```python
from build123d import *

# Parameters (mm, degrees)
F0_W     = 53
F0_H     = 10
F0_R     = 1.8
F1_DEPTH = 8
F2_R     = 1.8
F3_DEPTH = 5
F4_R     = 3


with BuildPart() as f1:
    # F0 (on Front) → F1 (new body)
    with BuildSketch(Plane.XZ):
        with Locations((-26.5, 5)):
            Rectangle(F0_W, F0_H)
        with Locations((-48.5, 5)):
            Circle(F0_R, mode=Mode.SUBTRACT)
        with Locations((-4.5, 5)):
            Circle(F0_R, mode=Mode.SUBTRACT)
        with Locations((-48.5, 5)):
            Circle(F0_R)
        with Locations((-4.5, 5)):
            Circle(F0_R)
    extrude(amount=F1_DEPTH)

    # F2 (on face) → F3 (cut)
    with BuildSketch(Plane(origin=(0, 0, 0), x_dir=(-1, 0, 0), z_dir=(0, 1, 0))):
        with Locations((4.5, 5)):
            Circle(F2_R)
        with Locations((48.5, 5)):
            Circle(F2_R)
    extrude(amount=-F3_DEPTH, mode=Mode.SUBTRACT)

    # F4
    f4_edges = [f1.edges().sort_by_distance(p)[0] for p in [
        (0, -4, 10),
        (0, -4, 0),
        (-53, -4, 10),
        (-53, -4, 0),
    ]]
    fillet(f4_edges, radius=F4_R)


solid = f1.part
```
Geometry: final body of the model. Coordinates: model frame, mm. A direction names the side the tool comes from. Give positions to 0.01 mm unless a question says otherwise; leave off trailing zeros. Loops run counter-clockwise (first coordinate to the right, second up) from the corner with the lowest first, then second, coordinate; pieces in that order, holes last. Notation, with made-up numbers: (35, 27) -> (52, 27) arc R28 ccw to (52, 62) -> close; hole circle Ø7 at (31, 36). An arc over 180 degrees is marked (long way). Return JSON: item names as keys, results as strings.
Item 1: Section C-C, the plane x = -48.5. Output: boundary loops of the cut face in (y, z).
Filled in:
{"outline": "(-8, 0) -> (0, 0) -> (0, 3.2) -> (-5, 3.2) -> (-5, 6.8) -> (0, 6.8) -> (0, 10) -> (-8, 10) -> close"}
Item 2: Section B-B, the plane z = 5. Output: boundary loops of the cut face in (x, y).
Filled in:
{"outline": "(-53, -8) -> (0, -8) -> (0, 0) -> (-2.7, 0) -> (-2.7, -5) -> (-6.3, -5) -> (-6.3, 0) -> (-46.7, 0) -> (-46.7, -5) -> (-50.3, -5) -> (-50.3, 0) -> (-53, 0) -> close"}
Item 3: Section A-A, the plane y = -3.75. Output: boundary loops of the cut face in (x, z), plus the area to 3 significant figures.
Filled in:
{"outline": "(-53, 3) arc R3 ccw to (-50, 0) -> (-3, 0) arc R3 ccw to (0, 3) -> (0, 7) arc R3 ccw to (-3, 10) -> (-50, 10) arc R3 ccw to (-53, 7) -> close; hole circle Ø3.6 at (-48.5, 5); hole circle Ø3.6 at (-4.5, 5)", "area": "502 mm^2"}
Item 4: Access query for faces 5 (the flat face through (-48, -5, 5)), 6 (the flat face through (0, -4, 5)). Directions: +Z, -Z, +X, -X, +Y, -Y. A direction counts if a zero-diameter tool reaches every point of the face in a straight line with its end or side. Return the directions, or none.
Filled in:
{"face 5": "+Y", "face 6": "+Z, -Z, +X, +Y, -Y"}
Item 5: Pin query (flat end, axial travel): P1, Ø1, axis at y = -6, z = 8, coming from the +X side. Return the tip coordinate at first contact, or that it passes through.
Filled in:
{"P1": "x = -0.04"}
Item 6: Mould query, pull axis Z, two halves, no side actions, for faces 1 (the flat face through (-4, -5, 5)), 2 (the flat face through (-27, -4, 0)), 3 (the flat face through (-27, -8, 5)), 4 (the cylindrical face through (-49.331, -2.465, 3.403)). Classes: released by +Z, released by -Z, zero draft, split by the parting line, or undercut.
Filled in:
{"face 1": "undercut", "face 2": "released by -Z", "face 3": "zero draft", "face 4": "undercut"}
Item 7: Line query: line 1 (Z direction, x = -48.5, y = -1.9); line 2 (X direction, y = -6.75, z = 9); line 3 (X direction, y = -5.75, z = 9.5). Output: solid intervals per line, ascending.
Filled in:
{"line 1": "0 to 3.2, 6.8 to 10", "line 2": "-52.24 to -0.76", "line 3": "-51.66 to -1.34"}
